Read the model definition and answer for the solid it produces. Units are mm, in the model's axes. Face numbers are marked on the shaded views. A direction names the side the tool comes from. Give positions to 0.01 mm unless a question says otherwise; leave off trailing zeros. Write each loop counter-clockwise with the first axis right and the second up, starting at its lowest first coordinate (ties: lowest second). Pieces come first, ordered by that corner, then holes.
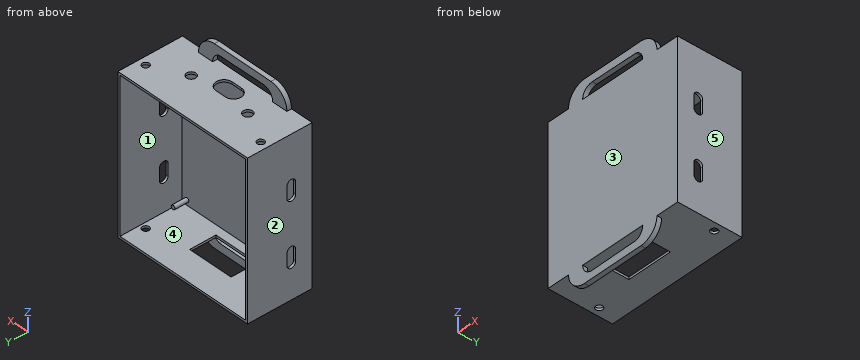
```python
from build123d import *

# Parameters (mm, degrees)
SKETCH_1_W               = 62
SKETCH_1_H               = 67
EXTRUDE_1_DEPTH          = 1
SKETCH_3_R               = 0.9
EXTRUDE_2_DEPTH          = 6
SKETCH_5_W               = 62
SKETCH_5_H               = 67
SKETCH_5_W_2             = 60
SKETCH_5_H_2             = 65
EXTRUDE_3_DEPTH          = 27
SKETCH_6_W               = 19.8
SKETCH_6_H               = 11.4
CUT_EXTRUDE_1_DEPTH      = 2
CUT_EXTRUDE_2_DEPTH      = 76.830402874
CUT_EXTRUDE_2_DEPTH_BACK = 76.830402874
CUT_EXTRUDE_3_DEPTH      = 2
SKETCH_8_3_R             = 2
CUT_EXTRUDE_4_DEPTH      = 10
SKETCH_9_R               = 1.5
CUT_EXTRUDE_5_DEPTH      = 79.955683773
EXTRUDE_4_DEPTH          = 2


with BuildPart() as part:
    # Sketch 1 → Extrude 1 (new body)
    with BuildSketch(Plane(origin=(0, 0, 0), x_dir=(1, 0, 0), z_dir=(0, 1, 0))):
        Rectangle(SKETCH_1_W, SKETCH_1_H)
    extrude(amount=EXTRUDE_1_DEPTH)

    # Sketch 3 → Extrude 2 (add)
    with BuildSketch(Plane(origin=(0, 1, 0), x_dir=(1, 0, 0), z_dir=(0, 1, 0))):
        with Locations(Location((27.75, -30.3, 0), (0, 0, 270))):
            Circle(SKETCH_3_R)
        with Locations(Location((27.75, 30.3, 0), (0, 0, 90))):
            Circle(SKETCH_3_R)
        with Locations(Location((-27.75, -30.3, 0), (0, 0, 90))):
            Circle(SKETCH_3_R)
        with Locations(Location((-27.75, 30.3, 0), (0, 0, 270))):
            Circle(SKETCH_3_R)
    extrude(amount=EXTRUDE_2_DEPTH)

    # Sketch 5 → Extrude 3 (add)
    with BuildSketch(Plane(origin=(0, 1, 0), x_dir=(1, 0, 0), z_dir=(0, 1, 0))):
        Rectangle(SKETCH_5_W, SKETCH_5_H)
        Rectangle(SKETCH_5_W_2, SKETCH_5_H_2, mode=Mode.SUBTRACT)
    extrude(amount=EXTRUDE_3_DEPTH)

    # Sketch 6 → Cut-Extrude 1 (cut)
    with BuildSketch(Plane(origin=(0, 0, -33.5), x_dir=(-1, 0, 0), z_dir=(0, 0, -1))):
        with Locations((0.1, 10.4)):
            Rectangle(SKETCH_6_W, SKETCH_6_H)
    extrude(amount=-CUT_EXTRUDE_1_DEPTH, mode=Mode.SUBTRACT)

    # Sketch 7 → Cut-Extrude 2 (cut, two sides: drawn at the far end of the back side and taken through both)
    with BuildSketch(Plane(origin=(31, 0, 0), x_dir=(0, 0, -1), z_dir=(1, 0, 0)).offset(-CUT_EXTRUDE_2_DEPTH_BACK)):
        with BuildLine():
            Line((-13.3, 10.9), (-8.3, 10.9))
            ThreePointArc((-8.3, 10.9), (-6.4, 9), (-8.3, 7.1))
            Line((-8.3, 7.1), (-13.3, 7.1))
            ThreePointArc((-13.3, 7.1), (-15.2, 9), (-13.3, 10.9))
        make_face()
        with BuildLine():
            Line((13.8, 10.9), (18.8, 10.9))
            ThreePointArc((18.8, 10.9), (20.7, 9), (18.8, 7.1))
            Line((18.8, 7.1), (13.8, 7.1))
            ThreePointArc((13.8, 7.1), (11.9, 9), (13.8, 10.9))
        make_face()
    extrude(amount=CUT_EXTRUDE_2_DEPTH + CUT_EXTRUDE_2_DEPTH_BACK, mode=Mode.SUBTRACT)

    # Sketch 8 → Cut-Extrude 3 (cut)
    with BuildSketch(Plane.XY.offset(33.5)):
        with BuildLine():
            Line((2.3, 11.5), (-2.2, 11.5))
            ThreePointArc((-2.2, 11.5), (-5.7, 8), (-2.2, 4.5))
            Line((-2.2, 4.5), (2.3, 4.5))
            ThreePointArc((2.3, 4.5), (5.8, 8), (2.3, 11.5))
        make_face()
    extrude(amount=-CUT_EXTRUDE_3_DEPTH, mode=Mode.SUBTRACT)

    # Sketch 8_3 → Cut-Extrude 4 (cut)
    with BuildSketch(Plane.XY.offset(33.5)):
        with Locations((-13.5, 12)):
            Circle(SKETCH_8_3_R)
        with Locations((13.6, 12)):
            Circle(SKETCH_8_3_R)
    extrude(amount=-CUT_EXTRUDE_4_DEPTH, mode=Mode.SUBTRACT)

    # Sketch 9 → Cut-Extrude 5 (cut, through all)
    with BuildSketch(Plane.XY.offset(33.5)):
        with Locations((-27.5, 19.1)):
            Circle(SKETCH_9_R)
        with Locations((27.5, 19.1)):
            Circle(SKETCH_9_R)
    extrude(amount=-CUT_EXTRUDE_5_DEPTH, mode=Mode.SUBTRACT)

    # Sketch 10 → Extrude 4 (add)
    with BuildSketch(Plane.XZ):
        with BuildLine():
            Line((14.370902848, -33.5), (21.143202049, -33.5))
            ThreePointArc((21.143202049, -33.5), (18.914555679, -38.964375793), (13.5, -41.311470647))
            Line((13.5, -41.311470647), (-13.5, -41.311470647))
            ThreePointArc((-13.5, -41.311470647), (-18.914555679, -38.964375793), (-21.143202049, -33.5))
            Line((-21.143202049, -33.5), (-14.370902848, -33.5))
            ThreePointArc((-14.370902848, -33.5), (-13.034801548, -36.725633878), (-9.80916767, -38.061735178))
            Line((-9.80916767, -38.061735178), (11.18974267, -37.847808701))
            ThreePointArc((11.18974267, -37.847808701), (13.490692176, -36.193660176), (14.370902848, -33.5))
        make_face()
        with BuildLine():
            Line((-21.143202049, 33.5), (-14.39209337, 33.5))
            Line((-14.39209337, 33.5), (-14.370902848, 33.5))
            ThreePointArc((-14.370902848, 33.5), (-13.034801548, 36.725633878), (-9.80916767, 38.061735178))
            Line((-9.80916767, 38.061735178), (11.18974267, 37.847808701))
            ThreePointArc((11.18974267, 37.847808701), (13.490692176, 36.193660176), (14.370902848, 33.5))
            Line((14.370902848, 33.5), (21.143202049, 33.5))
            ThreePointArc((21.143202049, 33.5), (18.914555679, 38.964375793), (13.5, 41.311470647))
            Line((13.5, 41.311470647), (-13.5, 41.311470647))
            ThreePointArc((-13.5, 41.311470647), (-18.914555679, 38.964375793), (-21.143202049, 33.5))
        make_face()
    extrude(amount=-EXTRUDE_4_DEPTH)


solid = part.part
```
Item 1: Find the intervals of material crossed by line 1 along Z through (x, y) = (-8.5, 24.75); line 2 along Y through (x, z) = (-27.5, -33); line 3 along X through (y, z) = (5.5, 17), in increasing order.
Result set:
line 1: z = -33.5 to -32.5, 32.5 to 33.5
line 2: y = 0 to 17.6, 20.6 to 28
line 3: x = -31 to -30, 30 to 31
Item 2: Each of these flat-tipped pins is pushed along its axis until it touches: pin 1 Ø8 at (x, y) = (9, 19) entering from -Z; pin 2 Ø2.5 at (x, y) = (-27.5, 19.1) entering from -Z; pin 3 Ø1.1 at (x, z) = (30.5, 11) entering from -Y; pin 4 Ø2.5 at (x, y) = (13.6, 12) entering from +Z. Where does it stop, or does it pass through?
Result set:
pin 1: stops at z = -33.5
pin 2: passes through
pin 3: stops at y = 0
pin 4: stops at z = -32.5
Item 3: Section A-A (y = 22.25) is taken. Write down the section's boundary in (x, z), and give its area (3 significant figures).
Result set:
outline: (-31, -33.5) - (31, -33.5) - (31, 33.5) - (-31, 33.5) - close; hole (-30, -32.5) - (30, -32.5) - (30, 32.5) - (-30, 32.5) - close
area: 254 mm2
Item 4: Section C-C (y = 3.5) is taken. Write down the section's boundary in (x, z), and give its area (3 significant figures).
Result set:
outline: (-31, -33.5) - (31, -33.5) - (31, 33.5) - (-31, 33.5) - close; circle Ø1.8 at (-27.75, -30.3); circle Ø1.8 at (-27.75, 30.3); circle Ø1.8 at (27.75, -30.3); circle Ø1.8 at (27.75, 30.3); hole (-30, -32.5) - (30, -32.5) - (30, 32.5) - (-30, 32.5) - close
area: 264 mm2
Item 5: Which of the six approach directions +Z, -Z, +X, -X, +Y, -Y give full straight-line access (tool end or side, diameter ignored) to the marked faces 1 and 2?
Result set:
face 1: +Y
face 2: +Z, -Z, -X, +Y, -Y
Item 6: Section D-D (x = -24.5) is taken. Write down the section's boundary in (y, z).
Result set:
outline: (0, -33.5) - (28, -33.5) - (28, -32.5) - (1, -32.5) - (1, 32.5) - (28, 32.5) - (28, 33.5) - (0, 33.5) - close
Item 7: Section B-B (z = 12) is taken. Write down the section's boundary in (x, y).
Result set:
outline: (-31, 0) - (31, 0) - (31, 7.1) - (30, 7.1) - (30, 1) - (-30, 1) - (-30, 7.1) - (-31, 7.1) - close; (-31, 10.9) - (-30, 10.9) - (-30, 28) - (-31, 28) - close; (30, 10.9) - (31, 10.9) - (31, 28) - (30, 28) - close
Item 8: Determine the mould class of the marked faces 3, 4 and 5 for opening direction X: pulls with the +X half, pulls with the -X half, needs draft (parallel to the pull), parting line crosses it, or undercut.
Result set:
face 3: needs draft
face 4: undercut
face 5: pulls with the +X half
